from build123d import *

# Parameters (mm, degrees)
BOSS_EXTRUDE1_DEPTH = 0.01
BOSS_EXTRUDE2_DEPTH = 0.64
CUT_EXTRUDE1_START  = 0.64
CUT_EXTRUDE1_DEPTH  = 0.32
SKETCH4_W           = 0.8
SKETCH4_H           = 2.25
BOSS_EXTRUDE3_DEPTH = 0.32


with BuildPart() as part:
    # Sketch1 → Revolve1 (revolve)
    with BuildSketch(Plane.XY):
        with BuildLine():
            Line((0, 5.5), (-2.3, 5.5))
            ThreePointArc((-2.3, 5.5), (-2.441421356, 5.441421356), (-2.5, 5.3))
            Line((-2.5, 5.3), (-2.5, 1.2))
            ThreePointArc((-2.5, 1.2), (-2.441421356, 1.058578644), (-2.3, 1))
            Line((-2.3, 1), (-2.3, 0.8))
            ThreePointArc((-2.3, 0.8), (-2.441421356, 0.741421356), (-2.5, 0.6))
            Line((-2.5, 0.6), (-2.5, 0))
            Line((-2.5, 0), (0, 0))
            Line((0, 0), (0, 5.5))
        make_face()
    revolve(axis=Axis((0, 8.082229881, 0), (0, -1, 0)))

    # Sketch2 → Boss-Extrude1 (add)
    with BuildSketch(Plane(origin=(0, 5.5, 0), x_dir=(1, 0, 0), z_dir=(0, 1, 0))):
        with BuildLine():
            Line((-1.962141687, 1.2), (1.962141687, 1.2))
            ThreePointArc((1.962141687, 1.2), (0, 2.3), (-1.962141687, 1.2))
        make_face()
    extrude(amount=BOSS_EXTRUDE1_DEPTH)

    # Sketch3 → Boss-Extrude2 (add)
    with BuildSketch(Plane(origin=(0, 0, 0), x_dir=(-1, 0, 0), z_dir=(0, -1, 0))):
        Polygon((1.589339828, -2.65), (2.65, -1.589339828), (2.65, 2.65), (-2.65, 2.65), (-2.65, -1.589339828), (-1.589339828, -2.65), align=None)
    extrude(amount=BOSS_EXTRUDE2_DEPTH)

    # Sketch3<3> → Cut-Extrude1 (cut)
    with BuildSketch(Plane(origin=(0, 0, 0), x_dir=(-1, 0, 0), z_dir=(0, -1, 0)).offset(CUT_EXTRUDE1_START)):
        with BuildLine():
            Line((0.4, 0.5), (0.4, 2.467792536))
            ThreePointArc((0.4, 2.467792536), (0, 2.5), (-0.4, 2.467792536))
            Line((-0.4, 2.467792536), (-0.4, 0.5))
            Line((-0.4, 0.5), (0.4, 0.5))
        make_face()
        with BuildLine():
            ThreePointArc((-0.4, -2.467792536), (0, -2.5), (0.4, -2.467792536))
            Line((0.4, -2.467792536), (0.4, -0.5))
            Line((0.4, -0.5), (-0.4, -0.5))
            Line((-0.4, -0.5), (-0.4, -2.467792536))
        make_face()
        with BuildLine():
            Line((0.4, 2.467792536), (0.4, 2.65))
            Line((0.4, 2.65), (-0.4, 2.65))
            Line((-0.4, 2.65), (-0.4, 2.467792536))
            ThreePointArc((-0.4, 2.467792536), (0, 2.5), (0.4, 2.467792536))
        make_face()
        with BuildLine():
            Line((-0.4, -2.65), (0.4, -2.65))
            Line((0.4, -2.65), (0.4, -2.467792536))
            ThreePointArc((0.4, -2.467792536), (0, -2.5), (-0.4, -2.467792536))
            Line((-0.4, -2.467792536), (-0.4, -2.65))
        make_face()
    extrude(amount=-CUT_EXTRUDE1_DEPTH, mode=Mode.SUBTRACT)

    # Sketch4 → Boss-Extrude3 (add)
    with BuildSketch(Plane.XZ.offset(0.32)):
        with Locations((0, -1.625)):
            Rectangle(SKETCH4_W, SKETCH4_H)
        with Locations((0, 1.625)):
            Rectangle(SKETCH4_W, SKETCH4_H)
    extrude(amount=BOSS_EXTRUDE3_DEPTH)


solid = part.part
Read the model definition and answer for the solid it produces. Units are mm, in the model's axes. A direction names the side the tool comes from. Round coordinates to 2 decimals unless told otherwise and drop trailing zeros. Order: outer loops, then holes, each group sorted by start corner. A loop starts at its lowest first (then second) coordinate and runs counter-clockwise, first axis right, second up.
1) Straight lines are drawn through the part: L1, parallel to Y at x = -1.25, z = -0.2; L2, parallel to Y at x = 2.3, z = 1.15; L3, parallel to Z at x = 0.3, y = 1.5. For each, find the intervals that lie inside material, in ascending order.
2) The part is cut by section C-C on y = 2.25. Write down the section's boundary in (x, z), plus the area to 3 significant figures.
3) The part is cut by section A-A on z = 0. Write down the section's boundary in (x, y).
4) For faces 1 (the face through (0, 5.5, 1)), 2 (the face through (0, -0.64, 0)), 3 (the face through (0.54, 0.3, 2.44)), determine the directions among +Z, -Z, +X, -X, +Y, -Y from which every point of the face is accessible in a straight line to the end or side of a thin tool.
5) Flat-ended cylindrical pins translate along their axes: pin 1 (1.6 mm diameter, centred on x = 0, z = 0, fed in from +Y); pin 2 (1.5 mm diameter, centred on y = 1.5, z = -1.5, fed in from +X). Find the tip coordinate at first contact, or state that the pin passes through.
Resolved:
1. L1: y = -0.64 to 5.5
1. L2: y = -0.64 to 0
1. L3: z = -2.48 to 2.48
2. outline: circle Ø5 at (0, 0)
2. area: 19.6 mm2
3. outline: (-2.65, -0.64) - (2.65, -0.64) - (2.65, 0) - (2.5, 0) - (2.5, 0.6) arc R0.2 ccw to (2.3, 0.8) - (2.3, 1) arc R0.2 ccw to (2.5, 1.2) - (2.5, 5.3) arc R0.2 ccw to (2.3, 5.5) - (-2.3, 5.5) arc R0.2 ccw to (-2.5, 5.3) - (-2.5, 1.2) arc R0.2 ccw to (-2.3, 1) - (-2.3, 0.8) arc R0.2 ccw to (-2.5, 0.6) - (-2.5, 0) - (-2.65, 0) - close
4. face 1: +Z, +X, -X, +Y
4. face 2: +Z, -Z, +X, -X, -Y
4. face 3: +Y
5. pin 1: stops at y = 5.5
5. pin 2: stops at x = 2.38
